```python
from build123d import *

# Parameters (mm, degrees)
ESTRUSIONE_ESTRUSIONE1_DEPTH = 4.5
NERVATURA1_START             = -4.55
NERVATURA1_DEPTH             = 9.1
ESTRUSIONE_ESTRUSIONE2_DEPTH = 7
TAGLIO_ESTRUSIONE1_DEPTH     = 3.3
ESTRUSIONE_ESTRUSIONE3_DEPTH = 2
FORO1_D                      = 3.2
FORO2_D                      = 3.2
SCHIZZO10_W                  = 29.5
SCHIZZO10_H                  = 2.3
SCHIZZO10_W_2                = 9.7
TAGLIO_ESTRUSIONE2_DEPTH     = 4.3
SCHIZZO11_W                  = 16.35
SCHIZZO11_H                  = 7.2
SCHIZZO11_W_2                = 16.05
SCHIZZO11_H_2                = 6.904461538
ESTRUSIONE_ESTRUSIONE4_DEPTH = 2
SCHIZZO12_R                  = 2.885572668
TAGLIO_ESTRUSIONE3_DEPTH     = 2
SCHIZZO15_W                  = 7.5
SCHIZZO15_H                  = 7.2
SCHIZZO15_R                  = 3.038054308
ESTRUSIONE_ESTRUSIONE5_DEPTH = 2


# Read off the part's stored shape, not the designer's step: Nervatura1
with BuildPart() as part:
    # Schizzo1 → Estrusione-Estrusione1 (new body)
    with BuildSketch(Plane.XY.offset(4.5)):
        Polygon((5.05, -9.992575631), (5.05, -6.5), (14.75, -6.5), (14.75, 6.5), (-14.75, 6.5), (-14.75, -6.5), (-5.05, -6.5), (-5.05, -9.992575631), align=None)
    extrude(amount=-ESTRUSIONE_ESTRUSIONE1_DEPTH)

    # Nervatura1 outline → Nervatura1 (add)
    with BuildSketch(Plane.YZ.offset(NERVATURA1_START)):
        Polygon((-4.296088186, 4.5), (-5.110000145, 7.951589572), (-9.866118458, 7.398410428), (-9.866118458, 4.5), align=None)
    extrude(amount=NERVATURA1_DEPTH)

    # Schizzo3 → Estrusione-Estrusione2 (add)
    with BuildSketch(Plane.XY.offset(4.5)):
        Polygon((-14.75, -6.5), (-14.75, 6.5), (14.75, 6.5), (14.75, -6.5), (5.05, -6.5), (5.05, -4.2), (-5.05, -4.2), (-5.05, -6.5), align=None)
    extrude(amount=ESTRUSIONE_ESTRUSIONE2_DEPTH)

    # Schizzo4 → Taglio-Estrusione1 (cut)
    with BuildSketch(Plane(origin=(0, 0, 0), x_dir=(-1, 0, 0), z_dir=(0, 0, -1))):
        Polygon((5.05, -9.992575631), (5.05, -6.5), (5.05, -6), (14.25, -6), (14.25, 6), (-14.25, 6), (-14.25, -6), (-5.05, -6), (-5.05, -6.5), (-5.05, -9.992575631), align=None)
    extrude(amount=-TAGLIO_ESTRUSIONE1_DEPTH, mode=Mode.SUBTRACT)

    # Schizzo5 → Estrusione-Estrusione3 (add)
    with BuildSketch(Plane(origin=(0, 0, 0), x_dir=(-1, 0, 0), z_dir=(0, 0, -1))):
        with BuildLine():
            Line((14.75, 3.75), (14.75, -3.75))
            Line((14.75, -3.75), (18.5, -3.75))
            ThreePointArc((18.5, -3.75), (22.25, 0), (18.5, 3.75))
            Line((18.5, 3.75), (14.75, 3.75))
        make_face()
        with BuildLine():
            Line((-14.75, -3.75), (-14.75, 3.75))
            Line((-14.75, 3.75), (-18.5, 3.75))
            ThreePointArc((-18.5, 3.75), (-22.25, 0), (-18.5, -3.75))
            Line((-18.5, -3.75), (-14.75, -3.75))
        make_face()
    extrude(amount=-ESTRUSIONE_ESTRUSIONE3_DEPTH)

    # Foro1 (through all)
    with Locations(Plane.XY.offset(2)):
        with Locations((18.5, 0)):
            Hole(FORO1_D / 2)

    # Foro2 (through all)
    with Locations(Plane.XY.offset(2)):
        with Locations((-18.5, 0)):
            Hole(FORO2_D / 2)

    # Schizzo10 → Taglio-Estrusione2 (cut)
    with BuildSketch(Plane.XY.offset(11.5)):
        with Locations((0, 5.35)):
            Rectangle(SCHIZZO10_W, SCHIZZO10_H)
        with Locations((9.9, -5.35)):
            Rectangle(SCHIZZO10_W_2, SCHIZZO10_H)
        with Locations((-9.9, -5.35)):
            Rectangle(SCHIZZO10_W_2, SCHIZZO10_H)
    extrude(amount=-TAGLIO_ESTRUSIONE2_DEPTH, mode=Mode.SUBTRACT)

    # Schizzo11 → Estrusione-Estrusione4 (add)
    with BuildSketch(Plane.XY.offset(11.5)):
        with Locations((5.825, 0)):
            Rectangle(SCHIZZO11_W, SCHIZZO11_H)
        with Locations((5.825, 0.002230769)):
            Rectangle(SCHIZZO11_W_2, SCHIZZO11_H_2, mode=Mode.SUBTRACT)
    extrude(amount=ESTRUSIONE_ESTRUSIONE4_DEPTH)

    # Schizzo12 → Taglio-Estrusione3 (cut)
    with BuildSketch(Plane.XY.offset(11.5)):
        with Locations(Location((9.75, 0, 0), (0, 0, 180))):
            Circle(SCHIZZO12_R)
    extrude(amount=-TAGLIO_ESTRUSIONE3_DEPTH, mode=Mode.SUBTRACT)

    # Schizzo13 → Rivoluzione1 (revolve)
    with BuildSketch(Plane(origin=(0, 0, 0), x_dir=(1, 0, 0), z_dir=(0, 1, 0)), mode=Mode.PRIVATE) as rivoluzione1_sk:
        with BuildLine():
            Line((12.635572668, -9.5), (9.75, -9.5))
            Line((9.75, -9.5), (9.75, -11.5))
            ThreePointArc((9.75, -11.5), (11.505457891, -10.951118249), (12.635572668, -9.5))
        make_face()
    revolve(rivoluzione1_sk.sketch.rotate(Axis((9.75, 0, 9.5), (0, 0, 1)), 180), axis=Axis((9.75, 0, 9.5), (0, 0, 1)))

    # Schizzo14 → Rivoluzione2 (revolve)
    with BuildSketch(Plane(origin=(0, 0, 0), x_dir=(1, 0, 0), z_dir=(0, 1, 0)), mode=Mode.PRIVATE) as rivoluzione2_sk:
        with BuildLine():
            Line((-7.211945692, -11.5), (-10.25, -11.5))
            Line((-10.25, -11.5), (-10.25, -13.5))
            ThreePointArc((-10.25, -13.5), (-8.431362187, -12.955116727), (-7.211945692, -11.5))
        make_face()
    revolve(rivoluzione2_sk.sketch.rotate(Axis((-10.25, 0, 11.5), (0, 0, 1)), 180), axis=Axis((-10.25, 0, 11.5), (0, 0, 1)))

    # Schizzo15 → Estrusione-Estrusione5 (add)
    with BuildSketch(Plane.XY.offset(11.5)):
        with Locations((-10.25, 0)):
            Rectangle(SCHIZZO15_W, SCHIZZO15_H)
        with Locations((-10.25, 0)):
            Circle(SCHIZZO15_R, mode=Mode.SUBTRACT)
    extrude(amount=ESTRUSIONE_ESTRUSIONE5_DEPTH)


solid = part.part
```
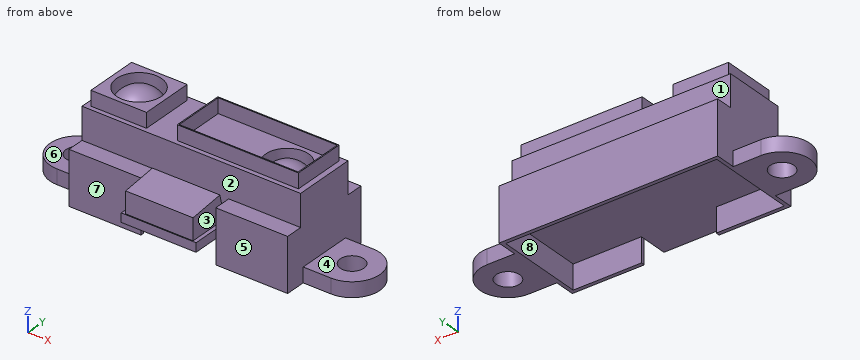
Could you check a few things on this model? Use its own coordinates, in mm. Face numbers are marked on the shaded views. A direction names the side the tool comes from. Coordinates: 2 decimals unless noted, no trailing zeros. Write each loop counter-clockwise with the first axis right and the second up, starting at its lowest first coordinate (ties: lowest second). Pieces come first, ordered by that corner, then holes. Notation, with made-up numbers: (-14, 80.5) -> (23, 80.5) arc R9 cw to (23, 97.5) -> close; hole circle Ø7 at (81.5, 48). An arc over 180 degrees is marked (long way). Return JSON: item names as keys, results as strings.
(1) Imagine slicing it at C-C, the plane x = -10.25. Please give me the cut outline in (y, z), then the cut area to 3 significant figures.
Numbers:
{"outline": "(-6.5, 0) -> (-6, 0) -> (-6, 3.3) -> (6, 3.3) -> (6, 0) -> (6.5, 0) -> (6.5, 7.2) -> (4.2, 7.2) -> (4.2, 11.5) -> (3.6, 11.5) -> (3.6, 13.5) -> (3.04, 13.5) -> (3.04, 11.5) arc R3.31 ccw to (-3.04, 11.5) -> (-3.04, 13.5) -> (-3.6, 13.5) -> (-3.6, 11.5) -> (-4.2, 11.5) -> (-4.2, 7.2) -> (-6.5, 7.2) -> close", "area": "101 mm2"}
(2) Which directions (+Z, -Z, +X, -X, +Y, -Y) give clear straight access to the entire face, cutting with the end or side of a thin tool? Please do the marked faces 1, 2, 3, 4 and 5.
Numbers:
{"face 1": "+Z, +X, -X, +Y", "face 2": "+Z", "face 3": "+Z, -Y", "face 4": "+Z, +X, +Y, -Y", "face 5": "+Z, -Z, +X, -Y"}
(3) I'm going to push flat-ended pins straight in: pin 1 (0.6 mm diameter, centred on x = 17.5, z = 1.5, fed in from -Y); pin 2 (2.5 mm diameter, centred on x = -8, y = -5, fed in from +Z); pin 3 (1.5 mm diameter, centred on x = 3, y = -5.5, fed in from +Z). Where does each tip first touch, or does it pass through?
Numbers:
{"pin 1": "stops at y = -3.75", "pin 2": "stops at z = 11.5", "pin 3": "stops at z = 7.95"}
(4) Imagine slicing it at B-B, the plane y = 5.25. Please give me the cut outline in (x, z).
Numbers:
{"outline": "(-14.75, 0) -> (-14.25, 0) -> (-14.25, 3.3) -> (14.25, 3.3) -> (14.25, 0) -> (14.75, 0) -> (14.75, 7.2) -> (-14.75, 7.2) -> close"}
(5) We'd pull the mould along Y, two halves only. Please class the marked faces 6, 7 and 8: +Y half, -Y half, draft (parallel to the pull), parting line (faces both ways), or undercut.
Numbers:
{"face 6": "draft", "face 7": "-Y half", "face 8": "undercut"}
(6) I need wall thicknesses on L1, parallel to X at y = -1.75, z = 2.25; L2, parallel to Y at x = 9.75, z = 10.8; L3, parallel to Y at x = -10.25, z = 12.5. Which ranges of each line are inside material? Lowest first, please.
Numbers:
{"L1": "x = -14.75 to -14.25, 14.25 to 14.75", "L2": "y = -4.2 to -2.89, -1.96 to 1.96, 2.89 to 4.2", "L3": "y = -3.6 to -3.04, -2.37 to 2.37, 3.04 to 3.6"}
(7) Imagine slicing it at A-A, the plane z = 1. Please give me the cut outline in (x, y), then the cut area to 3 significant figures.
Numbers:
{"outline": "(-18.5, -3.75) -> (-14.75, -3.75) -> (-14.75, -6.5) -> (-5.05, -6.5) -> (-5.05, -6) -> (-14.25, -6) -> (-14.25, 6) -> (14.25, 6) -> (14.25, -6) -> (5.05, -6) -> (5.05, -6.5) -> (14.75, -6.5) -> (14.75, -3.75) -> (18.5, -3.75) arc R3.75 ccw to (18.5, 3.75) -> (14.75, 3.75) -> (14.75, 6.5) -> (-14.75, 6.5) -> (-14.75, 3.75) -> (-18.5, 3.75) arc R3.75 ccw to start; hole circle Ø3.2 at (-18.5, 0); hole circle Ø3.2 at (18.5, 0)", "area": "121 mm2"}
(8) Imagine slicing it at D-D, the plane z = 5.25. Please give me the cut outline in (x, y).
Numbers:
{"outline": "(-14.75, -6.5) -> (-5.05, -6.5) -> (-5.05, -4.2) -> (5.05, -4.2) -> (5.05, -6.5) -> (14.75, -6.5) -> (14.75, 6.5) -> (-14.75, 6.5) -> close; (-4.55, -9.87) -> (4.55, -9.87) -> (4.55, -4.47) -> (-4.55, -4.47) -> close"}
